from build123d import *

# Parameters (mm, degrees)
F0_W     = 381
F0_H     = 609.6
F1_DEPTH = 876.3
F2_W     = 381
F2_H     = 88.9
F3_DEPTH = 88.9
F4_T     = -12.7
F5_DEPTH = 88.9
F6_W     = 381
F6_H     = 787.4
F7_DEPTH = 12.7


with BuildPart() as f1:
    # F0 (on Top) → F1 (new body)
    with BuildSketch(Plane.XY):
        with Locations((190.5, -304.8)):
            Rectangle(F0_W, F0_H)
    extrude(amount=F1_DEPTH)

    # F2 (on face) → F3 (cut)
    with BuildSketch(Plane.XZ.offset(609.6)):
        with Locations((190.5, 44.45)):
            Rectangle(F2_W, F2_H)
    extrude(amount=-F3_DEPTH, mode=Mode.SUBTRACT)

    # F4
    f4_openings = [f1.faces().sort_by_distance(p)[0] for p in [
        (190.5, -609.6, 482.6),
    ]]
    offset(amount=F4_T, openings=f4_openings, kind=Kind.INTERSECTION)

    # F5 (add, through all): a face of the model
    f5_faces = [f1.faces().sort_by_distance(p)[0] for p in [
        (190.5, -260.35, 12.7),
    ]]
    extrude(f5_faces, amount=F5_DEPTH)

    # F6 (on face) → F7 (join)
    with BuildSketch(Plane.XZ.offset(609.6)):
        with Locations((190.5, 482.6)):
            Rectangle(F6_W, F6_H)
        Polygon((342.9, 101.6), (38.1, 101.6), (12.7, 101.6), (12.7, 863.6), (368.3, 863.6), (368.3, 101.6), align=None, mode=Mode.SUBTRACT)
        Polygon((38.1, 101.6), (38.1, 838.2), (342.9, 838.2), (342.9, 101.6), (368.3, 101.6), (368.3, 863.6), (12.7, 863.6), (12.7, 101.6), align=None)
    extrude(amount=-F7_DEPTH)


solid = f1.part
The listing builds one solid part. Answer for the finished solid, in the listing's coordinates (mm). A direction names the side the tool comes from. Coordinates: 2 decimals unless noted, no trailing zeros. Write each loop counter-clockwise with the first axis right and the second up, starting at its lowest first coordinate (ties: lowest second). Pieces come first, ordered by that corner, then holes. Notation, with made-up numbers: (-33.5, 26) - (-27.5, 26) arc R19 ccw to (-27.5, 42) - close; hole circle Ø8 at (-22.75, 37). An arc over 180 degrees is marked (long way). Answer as CSV lines item,"result".
1. Straight lines are drawn through the part: line 1 (Z direction, x = 335, y = -148); line 2 (X direction, y = -265, z = 370); line 3 (Y direction, x = 350, z = 239.5). For each, find the intervals that lie inside material, in ascending order. Write a range as [from, to].
Computed values:
line 1,"z = [0, 101.6], [863.6, 876.3]"
line 2,"x = [0, 12.7], [368.3, 381]"
line 3,"y = [-609.6, -596.9], [-12.7, 0]"
2. Find section A-A (x = 25.5). Give the vertices of the cut face in (y, z).
Computed values:
outline,"(-609.6, 88.9) - (-520.7, 88.9) - (-520.7, 0) - (0, 0) - (0, 876.3) - (-609.6, 876.3) - close; hole (-596.9, 101.6) - (-12.7, 101.6) - (-12.7, 863.6) - (-596.9, 863.6) - close"
3. A tool of negligible diameter and unlimited length cuts with its end or side. For faces 1 (the flat face through (188, -12.7, 477)), 2 (the flat face through (188, 0, 432)), 3 (the flat face through (188, -566, 88.9)), from which of +Z, -Z, +X, -X, +Y, -Y can it reach the whole face along a straight path? Write none if from no direction.
Computed values:
face 1,"none"
face 2,"+Z, -Z, +X, -X, +Y"
face 3,"-Z, +X, -X, -Y"
4. Find section B-B (y = -127). Give the vertices of the cut face in (x, z).
Computed values:
outline,"(0, 0) - (381, 0) - (381, 876.3) - (0, 876.3) - close; hole (12.7, 101.6) - (368.3, 101.6) - (368.3, 863.6) - (12.7, 863.6) - close"
5. Given P1, Ø4, axis at x = 215, y = -602.5, coming from the -Z side; P2, Ø6, axis at y = -236, z = 674.5, coming from the -X side; P3, Ø6, axis at x = 153.5, z = 157, coming from the -Y side, each flat-ended and moving along its own axis, determine where each tip first touches the part or whether it passes through.
Computed values:
P1,"stops at z = 88.9"
P2,"stops at x = 0"
P3,"stops at y = -12.7"
6. Determine the mould class of faces 4 (the flat face through (188, -520.7, 45)), 5 (the flat face through (368.3, -309, 477)), 6 (the flat face through (188, -257, 0)), 7 (the flat face through (12.7, -309, 477)) for opening direction Z: +Z half, -Z half, draft (parallel to the pull), parting line (faces both ways), or undercut.
Computed values:
face 4,"draft"
face 5,"undercut"
face 6,"-Z half"
face 7,"undercut"
7. Find section C-C (z = 429). Give the vertices of the cut face in (x, y), plus the area to 3 significant figures.
Computed values:
outline,"(0, -609.6) - (38.1, -609.6) - (38.1, -596.9) - (12.7, -596.9) - (12.7, -12.7) - (368.3, -12.7) - (368.3, -596.9) - (342.9, -596.9) - (342.9, -609.6) - (381, -609.6) - (381, 0) - (0, 0) - close"
area,"20,600 mm²"
8. Find section D-D (x = 100). Give the vertices of the cut face in (y, z).
Computed values:
outline,"(-609.6, 88.9) - (-520.7, 88.9) - (-520.7, 0) - (0, 0) - (0, 876.3) - (-609.6, 876.3) - (-609.6, 838.2) - (-596.9, 838.2) - (-596.9, 863.6) - (-12.7, 863.6) - (-12.7, 101.6) - (-609.6, 101.6) - close"
